from build123d import *

# Parameters (mm, degrees)
SKETCH2_W            = 323.85
SKETCH2_H            = 22.86
SKETCH2_W_2          = 304.8
SKETCH2_H_2          = 12.7
BOSS_EXTRUDE1_DEPTH  = 5.08
CUT_EXTRUDE1_DEPTH   = 6.35
SKETCH4_W            = 6.35
SKETCH4_H            = 12.7
BOSS_EXTRUDE2_DEPTH  = 2.54
CUT_EXTRUDE3_DEPTH   = 325.091459005
CHAMFER5_SIZE        = 6.5287398
CHAMFER5_SIZE_2      = 4.571472823
BOSS_EXTRUDE4_DEPTH  = 6.35
CUT_EXTRUDE5_DEPTH   = 2.8575
M3_CLEARANCE_HOLE1_D = 3.2


with BuildPart() as part:
    # Sketch2 → Boss-Extrude1 (new body)
    with BuildSketch(Plane(origin=(0, 0, 0), x_dir=(1, 0, 0), z_dir=(0, 1, 0))):
        with Locations((-3.175, 0)):
            Rectangle(SKETCH2_W, SKETCH2_H)
        Rectangle(SKETCH2_W_2, SKETCH2_H_2, mode=Mode.SUBTRACT)
    extrude(amount=BOSS_EXTRUDE1_DEPTH)

    # Sketch3 → Cut-Extrude1 (cut)
    with BuildSketch(Plane.ZY.offset(165.1)):
        Polygon((-2.54, 5.08), (2.54, 5.08), (6.35, 0), (-6.35, 0), align=None)
    extrude(amount=-CUT_EXTRUDE1_DEPTH, mode=Mode.SUBTRACT)

    # Sketch4 → Boss-Extrude2 (add)
    with BuildSketch(Plane(origin=(0, 0, 0), x_dir=(1, 0, 0), z_dir=(0, 1, 0))):
        Rectangle(SKETCH4_W, SKETCH4_H)
    extrude(amount=BOSS_EXTRUDE2_DEPTH)

    # Sketch6 → Cut-Extrude3 (cut, through all)
    with BuildSketch(Plane(origin=(158.75, 0, 0), x_dir=(0, 0, -1), z_dir=(1, 0, 0))):
        Polygon((-11.43, 5.08), (-6.35, 0), (-11.43, 0), align=None)
        Polygon((11.43, 0), (6.35, 0), (11.43, 5.08), align=None)
    extrude(amount=-CUT_EXTRUDE3_DEPTH, mode=Mode.SUBTRACT)

    # Chamfer5
    # the kernel refuses this chamfer: 6.5287398, 4.571472823 mm, written as the material it takes off along each edge
    with BuildSketch(Plane(origin=(-152.4, 0, -6.35), x_dir=(0.02220967419845904, 0.9997533347641299, 0), z_dir=(0, 0, 1))) as chamfer5_piece_1:
        Polygon((CHAMFER5_SIZE * 0.999753334764, CHAMFER5_SIZE * 0.0222096741985), (-CHAMFER5_SIZE_2 * 0.0222096741983, CHAMFER5_SIZE_2 * 0.999753334758), (0, 0), align=None)
    extrude(amount=12.7, mode=Mode.SUBTRACT)

    # Sketch8 → Boss-Extrude4 (add, symmetric)
    with BuildSketch(Plane.XY):
        with BuildLine():
            Line((152.4, 0), (152.4, -6.35))
            ThreePointArc((152.4, -6.35), (155.575, -9.525), (158.75, -6.35))
            Line((158.75, -6.35), (158.75, 0))
            Line((158.75, 0), (152.4, 0))
        make_face()
    extrude(amount=BOSS_EXTRUDE4_DEPTH, both=True)

    # Sketch8<2> → Cut-Extrude5 (cut, symmetric)
    with BuildSketch(Plane.XY):
        with BuildLine():
            Line((152.4, 0), (152.4, -6.35))
            ThreePointArc((152.4, -6.35), (155.575, -9.525), (158.75, -6.35))
            Line((158.75, -6.35), (158.75, 0))
            Line((158.75, 0), (152.4, 0))
        make_face()
    extrude(amount=CUT_EXTRUDE5_DEPTH, both=True, mode=Mode.SUBTRACT)

    # M3 Clearance Hole1 (through all)
    with Locations(Plane.XY.offset(6.35)):
        with Locations((155.575, -6.35)):
            Hole(M3_CLEARANCE_HOLE1_D / 2)


solid = part.part
Design review of the part built by this model. Coordinates are the model's own, in mm. A direction names the side the tool comes from. Round coordinates to 2 decimals unless told otherwise and drop trailing zeros. Loops run counter-clockwise (first coordinate to the right, second up) from the corner with the lowest first, then second, coordinate; pieces in that order, holes last. Notation, with made-up numbers: (-30, 84) - (3, 84) arc R14 cw to (3, 108) - close; hole circle Ø4 at (-17.5, 77.25). An arc over 180 degrees is marked (long way). One line per item, written item: value. Start each with the question number.
1) Consider section A-A on x = 52. Give the boundary of the cut face in (y, z).
2) For faces 1 (the flat face through (-155.168, 2.576, -0.089)), 2 (the flat face through (156, -4, 2.858)), 3 (the flat face through (-162, 2.6, 4.4)), 4 (the flat face through (152.4, 1, 0)), list the 3-axis set-ups (+Z, -Z, +X, -X, +Y, -Y) from which the entire face can be reached by the end or side of a thin tool; tool diameter is ignored.
3) To check wall thickness, follow L1, parallel to X at y = 0.5, z = 0.75 (3 decimals); L2, parallel to X at y = 0.25, z = 1 (3 decimals); L3, parallel to X at y = -4.25, z = -3.75. State the ranges of each line that lie inside material, in increasing order. Write a range as from..to.
4) Draft analysis for pull direction Z (two halves, no side actions). For faces 5 (the flat face through (-165.1, 4, 7)), 6 (the flat face through (0, 2.54, 0)), 7 (the flat face through (-0.91, 2.5, -8.85)), state which applies: +Z half, -Z half, draft (parallel to the pull), parting line (faces both ways), or undercut.
5) Insertion check: pin 1 Ø5 at (x, y) = (156.5, -5.5) entering from +Z; pin 2 Ø0.5 at (x, z) = (-157.5, 0) entering from -Y; pin 3 Ø5 at (x, y) = (47.5, 2.5) entering from +Z. Each pin has a flat end and moves straight along its axis. Give the tip position at first contact, or say it passes through.
Reported:
1. outline: (0, -6.35) - (5.08, -11.43) - (5.08, -6.35) - close; (0, 6.35) - (5.08, 6.35) - (5.08, 11.43) - close
2. face 1: -Y
2. face 2: +X, -X, -Y
2. face 3: -X, -Y
2. face 4: +Y, -Y
3. L1: x = -158.75..-156.621, -3.175..3.175, 152.4..158.75
3. L2: x = -158.75..-156.796, -3.175..3.175, 152.4..158.75
3. L3: x = 152.4..158.75
4. face 5: draft
4. face 6: undercut
4. face 7: -Z half
5. pin 1: stops at z = 6.35
5. pin 2: stops at y = 0
5. pin 3: stops at z = 11.35
